For this review, use the dimensioned drawing (mm, ordinates from the lowest corner) and the shaded views. Coordinates: 2 decimals unless noted, no trailing zeros. Write each loop counter-clockwise with the first axis right and the second up, starting at its lowest first coordinate (ties: lowest second). Pieces come first, ordered by that corner, then holes. Notation, with made-up numbers: M -15.5,3.25 L -11.5,3.25 A20 cw -11.5,39.25 Z; hole C 40,-10 d5. An arc over 180 degrees is marked long. Return JSON: item names as keys, results as strings.
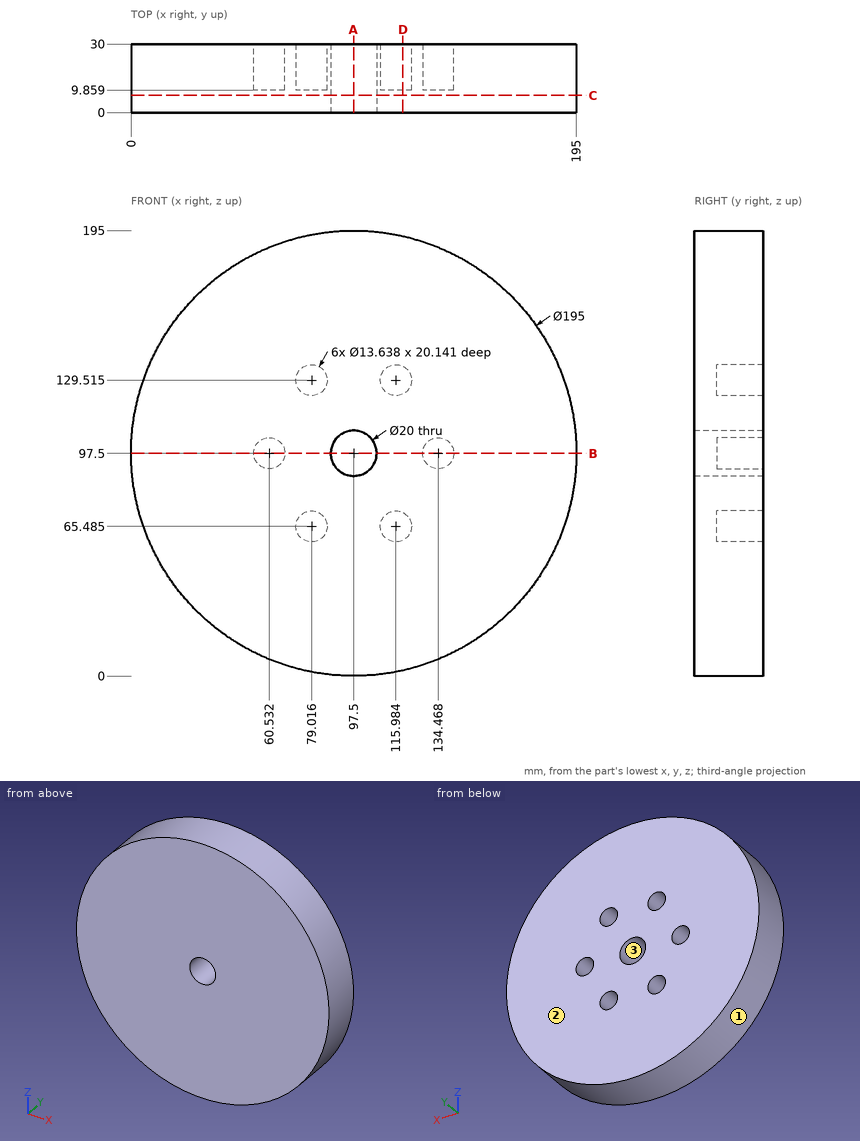
1. Clearance check with flat-ended pins moving along their axes: pin 1 Ø4 at (x, z) = (80, 126.5) entering from +Y; pin 2 Ø10 at (y, z) = (19, 67.5) entering from -X; pin 3 Ø1 at (x, y) = (136, 12.5) entering from +Z. State where each tip first meets the part, or that it passes through.
Checks:
{"pin 1": "y = 9.86", "pin 2": "x = 3.26", "pin 3": "z = 187.29"}
2. We need section C-C (y = 7.5). State the section outline as (x, z) points, plus the area to 3 significant figures.
Checks:
{"outline": "C 97.5,97.5 d195; hole C 97.5,97.5 d20", "area": "29,600 mm2"}
3. Wall thickness on L1, parallel to X at y = 15.75, z = 97.5; L2, parallel to Z at x = 74.5, y = 18.5 (1 decimal); L3, parallel to Y at x = 115.5, z = 59: over which ranges is each line inside the solid? List them lowest first. Write a range as from..to.
Checks:
{"L1": "0..53.71, 67.35..87.5, 107.5..127.65, 141.29..195", "L2": "2.8..60.4, 70.6..124.4, 134.6..192.2", "L3": "0..9.86"}
4. We need section A-A (x = 97.5). State the section outline as (y, z) points.
Checks:
{"outline": "M 0,0 L 30,0 L 30,87.5 L 0,87.5 Z; M 0,107.5 L 30,107.5 L 30,195 L 0,195 Z"}
5. We need section D-D (x = 119). State the section outline as (y, z) points.
Checks:
{"outline": "M 0,2.4 L 30,2.4 L 30,59.37 L 9.86,59.37 L 9.86,71.6 L 30,71.6 L 30,123.4 L 9.86,123.4 L 9.86,135.63 L 30,135.63 L 30,192.6 L 0,192.6 Z"}
6. We need section B-B (z = 97.5). State the section outline as (x, y) points.
Checks:
{"outline": "M 0,0 L 87.5,0 L 87.5,30 L 67.35,30 L 67.35,9.86 L 53.71,9.86 L 53.71,30 L 0,30 Z; M 107.5,0 L 195,0 L 195,30 L 141.29,30 L 141.29,9.86 L 127.65,9.86 L 127.65,30 L 107.5,30 Z"}
7. Draft analysis for pull direction X (two halves, no side actions). For the marked faces 1, 2 and 3, state which applies: +X half, -X half, draft (parallel to the pull), parting line (faces both ways), or undercut.
Checks:
{"face 1": "parting line", "face 2": "draft", "face 3": "undercut"}
